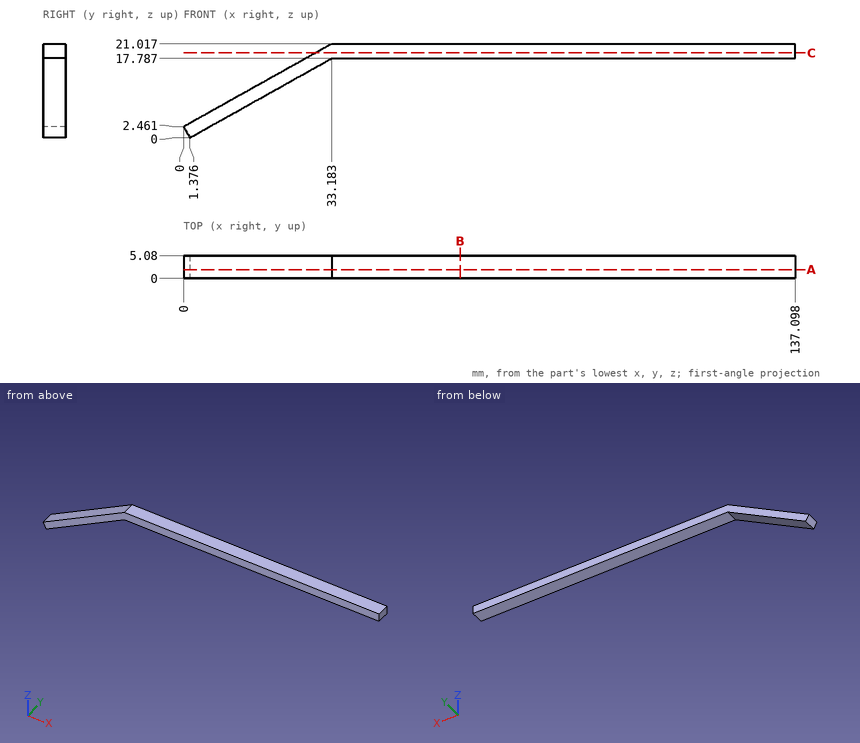
Design review of the part shown in the three views and the two pictorial views. Dimensions are in mm from the part's minimum x, y and z. Coordinates: 2 decimals unless noted, no trailing zeros. Order: outer loops, then holes, each group sorted by start corner. A loop starts at its lowest first (then second) coordinate and runs counter-clockwise, first axis right, second up.
1) Take a section at B-B, the plane x = 62. Give the boundary of the cut face in (y, z), and give its area (3 significant figures).
2) Wall thickness on line 1 along Z through (x, y) = (59, 0.6); line 2 along X through (y, z) = (0.9, 20.25) (1 decimal); line 3 along X through (y, z) = (2.7, 5.75) (1 decimal): over which ranges is each line inside the solid? List them lowest first.
3) Take a section at C-C, the plane z = 19. Give the boundary of the cut face in (x, y).
4) Take a section at A-A, the plane y = 1.95. Give the boundary of the cut face in (x, z).
5) Clearance check with flat-ended pins moving along their axes: pin 1 (2.5 mm diameter, centred on x = 109, y = 3.5, fed in from -Z); pin 2 (2 mm diameter, centred on y = 1.5, z = 13.5, fed in from -X) (1 decimal); pin 3 (2 mm diameter, centred on y = 2.5, z = 5.5, fed in from +X). State where each tip first meets the part, or that it passes through.
Returned:
1. outline: (0, 17.79) - (5.08, 17.79) - (5.08, 21.02) - (0, 21.02) - close
1. area: 16.4 mm2
2. line 1: z = 17.79 to 21.02
2. line 2: x = 31.8 to 137.1
2. line 3: x = 5.9 to 11.7
3. outline: (29.58, 0) - (137.1, 0) - (137.1, 5.08) - (29.58, 5.08) - close
4. outline: (0, 2.46) - (1.38, 0) - (33.18, 17.79) - (137.1, 17.79) - (137.1, 21.02) - (33.18, 21.02) - close
5. pin 1: stops at z = 17.79
5. pin 2: stops at x = 18
5. pin 3: stops at x = 13
